```python
from build123d import *

# Parameters (mm, degrees)
SZKIC1_W                    = 1000
SZKIC1_H                    = 173.21
SZKIC1_R                    = 7
DODANIE_WYCI_GNI_CIE1_DEPTH = 10
SZKIC3_W                    = 1000
SZKIC3_H                    = 10
DODANIE_WYCI_GNI_CIE3_DEPTH = 20
SZKIC4_W                    = 1000
SZKIC4_H                    = 20
DODANIE_WYCI_GNI_CIE4_DEPTH = 2080
SZKIC5_W                    = 1000
SZKIC5_H                    = 50
DODANIE_WYCI_GNI_CIE5_DEPTH = 500
SZKIC6_W                    = 1000
SZKIC6_H                    = 30
DODANIE_WYCI_GNI_CIE6_DEPTH = 1990
SZYK_LINIOWY1_COUNT         = 2
SZYK_LINIOWY1_PITCH         = 250


with BuildPart() as part:
    # Szkic1 → Dodanie-wyciągnięcie1 (new body)
    with BuildSketch(Plane.XY):
        Rectangle(SZKIC1_W, SZKIC1_H)
        with Locations((-482.5, 66.605)):
            Circle(SZKIC1_R, mode=Mode.SUBTRACT)
        with Locations(Location((482.5, 66.605, 0), (0, 0, 180))):
            Circle(SZKIC1_R, mode=Mode.SUBTRACT)
        with Locations(Location((-482.5, -66.605, 0), (0, 0, 180))):
            Circle(SZKIC1_R, mode=Mode.SUBTRACT)
        with Locations((482.5, -66.605)):
            Circle(SZKIC1_R, mode=Mode.SUBTRACT)
    dodanie_wyci_gni_cie1 = extrude(amount=DODANIE_WYCI_GNI_CIE1_DEPTH)

    # Szkic3 → Dodanie-wyciągnięcie3 (add)
    with BuildSketch(Plane(origin=(0, 86.605, 0), x_dir=(1, 0, 0), z_dir=(0, 1, 0))):
        with Locations((0, -5)):
            Rectangle(SZKIC3_W, SZKIC3_H)
    extrude(amount=DODANIE_WYCI_GNI_CIE3_DEPTH)

    # Szkic4 → Dodanie-wyciągnięcie4 (add)
    with BuildSketch(Plane.XY.offset(10)):
        with Locations((0, 96.605)):
            Rectangle(SZKIC4_W, SZKIC4_H)
    extrude(amount=DODANIE_WYCI_GNI_CIE4_DEPTH)

    # Lustro1: Dodanie-wyciągnięcie1 across plane
    add(dodanie_wyci_gni_cie1.mirror(Plane(origin=(0, 0, 1045), x_dir=(1, 0, 0), z_dir=(0, 0, -1))))

    # Szkic5 → Dodanie-wyciągnięcie5 (add)
    with BuildSketch(Plane(origin=(0, 106.605, 0), x_dir=(1, 0, 0), z_dir=(0, 1, 0))):
        with Locations((0, -2065)):
            Rectangle(SZKIC5_W, SZKIC5_H)
        with Locations((0, -25)):
            Rectangle(SZKIC5_W, SZKIC5_H)
    extrude(amount=DODANIE_WYCI_GNI_CIE5_DEPTH)

    # Szkic6 → Dodanie-wyciągnięcie6 (add)
    with BuildSketch(Plane(origin=(0, 0, 2040), x_dir=(-1, 0, 0), z_dir=(0, 0, -1))):
        with Locations((0, 341.605)):
            Rectangle(SZKIC6_W, SZKIC6_H)
    dodanie_wyci_gni_cie6 = extrude(amount=DODANIE_WYCI_GNI_CIE6_DEPTH)

    # Szyk liniowy1: Dodanie-wyciągnięcie6 ×2
    with Locations(*[(0, i * SZYK_LINIOWY1_PITCH, 0) for i in range(1, SZYK_LINIOWY1_COUNT)]):
        add(dodanie_wyci_gni_cie6)


solid = part.part
```
CAD build for the part. Positions are in the model's coordinates, mm. A direction names the side the tool comes from. Coordinates: 2 decimals unless noted, no trailing zeros. Write each loop counter-clockwise with the first axis right and the second up, starting at its lowest first coordinate (ties: lowest second). Pieces come first, ordered by that corner, then holes.
(1) Two-plate mould, pull along Y, no slides. Class faces 4 (the face through (-7, -1, 10)), 5 (the face through (-7, 465, 2040)), 6 (the face through (-7, 86.605, 1031)), 7 (the face through (-7, 465, 50)): +Y half, -Y half, draft (parallel to the pull), parting line (faces both ways), or undercut.
(2) Cut at C-C, the plane x = -398. List the corners of the cut face in (y, z) (3 decimals), and give its area (3 significant figures).
(3) Cut at B-B, the plane y = -38.5. List the corners of the cut face in (x, z), and give its area (3 significant figures).
(4) Drill centre lines: probe 1 along Y at (x, z) = (351.5, 480) (3 decimals); probe 2 along Y at (x, z) = (-482, 2086) (3 decimals); probe 3 along Z at (x, y) = (-2, 288). Where is each one in solid material? Low to high.
(5) Flat gauge pin, fed straight in: pin 1 (1 mm diameter, centred on x = 24, z = 1374, fed in from -Y) (3 decimals). Where does the tip first touch, or does it go through?
(6) 3-axis set-ups, long thin cutter, end or side, ignore diameter. For faces 1 (the face through (7, 326.605, 1059)), 2 (the face through (500, 335, 1050)), 3 (the face through (-7, 1, 2080)): which of +Z, -Z, +X, -X, +Y, -Y reach the whole face in a straight line?
(7) Cut at A-A, the plane z = 1876. List the corners of the cut face in (x, y) (3 decimals).
(8) Cut at D-D, the plane y = 230.5. List the corners of the cut face in (x, z), and give its area (3 significant figures).
Geometry says:
1. face 4: draft
1. face 5: undercut
1. face 6: -Y half
1. face 7: undercut
2. outline: (-86.605, 0) - (606.605, 0) - (606.605, 2090) - (-86.605, 2090) - (-86.605, 2080) - (86.605, 2080) - (86.605, 10) - (-86.605, 10) - close; hole (106.605, 50) - (326.605, 50) - (326.605, 2040) - (106.605, 2040) - close; hole (356.605, 50) - (576.605, 50) - (576.605, 2040) - (356.605, 2040) - close
2. area: 215,000 mm2
3. outline: (-500, 0) - (500, 0) - (500, 10) - (-500, 10) - close; (-500, 2080) - (500, 2080) - (500, 2090) - (-500, 2090) - close
3. area: 20,000 mm2
4. probe 1: y = 86.605 to 106.605, 326.605 to 356.605, 576.605 to 606.605
4. probe 2: y = -86.605 to -73.587, -59.623 to 59.623, 73.587 to 606.605
4. probe 3: z = 0 to 50, 2040 to 2090
5. pin 1: stops at y = 86.605
6. face 1: +X, -X
6. face 2: +Z, -Z, +X, +Y, -Y
6. face 3: +X, -X, -Y
7. outline: (-500, 86.605) - (500, 86.605) - (500, 106.605) - (-500, 106.605) - close; (-500, 326.605) - (500, 326.605) - (500, 356.605) - (-500, 356.605) - close; (-500, 576.605) - (500, 576.605) - (500, 606.605) - (-500, 606.605) - close
8. outline: (-500, 0) - (500, 0) - (500, 50) - (-500, 50) - close; (-500, 2040) - (500, 2040) - (500, 2090) - (-500, 2090) - close
8. area: 100,000 mm2
